from build123d import *

# Parameters (mm, degrees)
SKETCH1_R           = 2.25
BOSS_EXTRUDE1_DEPTH = 10
FILLET1_R           = 5
SKETCH2_R           = 2
CUT_EXTRUDE1_DEPTH  = 24


with BuildPart() as part:
    # Sketch1 → Boss-Extrude1 (new body)
    with BuildSketch(Plane(origin=(0, 0, 0), x_dir=(1, 0, 0), z_dir=(0, 1, 0))):
        with BuildLine():
            Line((32, 7.25), (-32, 7.25))
            ThreePointArc((-32, 7.25), (-35.535533906, 5.785533906), (-37, 2.25))
            Line((-37, 2.25), (-37, -7.25))
            Line((-37, -7.25), (37, -7.25))
            Line((37, -7.25), (37, 2.25))
            ThreePointArc((37, 2.25), (35.535533906, 5.785533906), (32, 7.25))
        make_face()
        with Locations(Location((23, 0, 0), (0, 0, 270))):
            Circle(SKETCH1_R, mode=Mode.SUBTRACT)
        with Locations(Location((-23, 0, 0), (0, 0, 270))):
            Circle(SKETCH1_R, mode=Mode.SUBTRACT)
    extrude(amount=BOSS_EXTRUDE1_DEPTH)

    # Fillet1
    fillet1_edges = [part.edges().sort_by_distance(p)[0] for p in [
        (37, 5, 7.25),
        (-37, 5, 7.25),
    ]]
    fillet(fillet1_edges, radius=FILLET1_R)

    # Sketch2 → Cut-Extrude1 (cut)
    with BuildSketch(Plane(origin=(0, 0, -7.25), x_dir=(-1, 0, 0), z_dir=(0, 0, -1))):
        with Locations((-12, 5)):
            Circle(SKETCH2_R)
        with Locations((12, 5)):
            Circle(SKETCH2_R)
    extrude(amount=-CUT_EXTRUDE1_DEPTH, mode=Mode.SUBTRACT)


solid = part.part
Geometry: final body of the model. Coordinates: model frame, mm. Give positions to 0.01 mm unless a question says otherwise; leave off trailing zeros. Write each loop counter-clockwise with the first axis right and the second up, starting at its lowest first coordinate (ties: lowest second). Pieces come first, ordered by that corner, then holes. Notation, with made-up numbers: M 51,32 L 108,32 A8 ccw 108,43 Z; hole C 42.25,85 d8. An arc over 180 degrees is marked long. Answer in a Markdown table with one row per item. Add a question column.
(1) First-contact query: pin 1 (6 mm diameter, centred on y = 6.5, z = 5.5, fed in from -X). Flat tip, straight axial feed; report the tip coordinate or a pass-through.
(2) Section C-C on y = 5. Return loops of the section in (x, z).
(3) Section B-B on z = 0. Return loops of the section in (x, y), and give its area (3 significant figures).
(4) Mould query, pull axis Y, two halves, no side actions, for faces 1 (the flat face through (0, 5, 7.25)), 2 (the flat face through (-1, 0, 0)), 3 (the cylindrical face through (-10, 5, 0)). Classes: +Y half, -Y half, draft (parallel to the pull), parting line (faces both ways), or undercut.
(5) Section A-A on x = 12. Return loops of the section in (y, z), and give its area (3 significant figures).
(6) Section D-D on y = 8.5. Return loops of the section in (x, z).
(7) Ray query, line 1 (X direction, y = 7.5, z = 0); line 2 (Y direction, x = 12, z = -3.25); line 3 (X direction, y = 5.75, z = 4.75). Return the intervals inside material, ascending.
Result set:
| question | item | result |
|---|---|---|
| 1 | pin 1 | stops at x = -36.99 |
| 2 | outline | M -37,-2.25 A5 ccw -32,-7.25 L -14,-7.25 L -14,7.25 L -32,7.25 A5 ccw -37,2.25 Z; M -10,-7.25 L 10,-7.25 L 10,7.25 L -10,7.25 Z; M 14,-7.25 L 32,-7.25 A5 ccw 37,-2.25 L 37,2.25 A5 ccw 32,7.25 L 14,7.25 Z; hole C -23,0 d4.5; hole C 23,0 d4.5 |
| 3 | outline | M -37,0 L -25.25,0 L -25.25,10 L -37,10 Z; M -20.75,0 L 20.75,0 L 20.75,10 L -20.75,10 Z; M 25.25,0 L 37,0 L 37,10 L 25.25,10 Z; hole C -12,5 d4; hole C 12,5 d4 |
| 3 | area | 625 mm^2 |
| 4 | face 1 | draft |
| 4 | face 2 | -Y half |
| 4 | face 3 | undercut |
| 5 | outline | M 0,-7.25 L 3,-7.25 L 3,7.25 L 0,7.25 Z; M 7,-7.25 L 10,-7.25 L 10,7.25 L 7,7.25 Z |
| 5 | area | 87.0 mm^2 |
| 6 | outline | M -37,-2.25 A5 ccw -32,-7.25 L 32,-7.25 A5 ccw 37,-2.25 L 37,2.25 A5 ccw 32,7.25 L -32,7.25 A5 ccw -37,2.25 Z; hole C -23,0 d4.5; hole C 23,0 d4.5 |
| 7 | line 1 | x = -37 to -25.25, -20.75 to 20.75, 25.25 to 37 |
| 7 | line 2 | y = 0 to 3, 7 to 10 |
| 7 | line 3 | x = -36.33 to -13.85, -10.15 to 10.15, 13.85 to 36.33 |
